Model file for the job. Use its own axes, mm. Face numbers are marked on the shaded views. Coordinates: 2 decimals unless noted, no trailing zeros. Write each loop counter-clockwise with the first axis right and the second up, starting at its lowest first coordinate (ties: lowest second). Pieces come first, ordered by that corner, then holes. Notation, with made-up numbers: M 0,46 L 21,46 A27 cw 21,62 Z; hole C 86,4.25 d4. An arc over 180 degrees is marked long. Put each result on its own line as item: value. Start each with the question number.
Q1. Cut at B-B (y = 21.5). Write the cut outline in (x, z).
Q2. Drop flat-ended pins along their axis: pin 1 (10 mm diameter, centred on y = 10.5, z = -65, fed in from +X); pin 2 (5 mm diameter, centred on x = 0.5, z = -72, fed in from +Y). Give the stop position or say it passes through.
Q3. Pull direction X, two halves, no side cores. Call the marked faces 1, 2 and 3: pulls with the +X half, pulls with the -X half, needs draft (parallel to the pull), parting line crosses it, or undercut.
Q4. Cut at C-C (x = -4). Write the cut outline in (y, z).
Q5. Cut at A-A (z = -57). Write the cut outline in (x, y).
Q6. Drill centre lines: line 1 along X through (y, z) = (9, -53); line 2 along Y through (x, z) = (1, -37); line 3 along X through (y, z) = (2, -64.5). Where is each one in solid material? Low to high.
Q7. Cut at D-D (z = -47.5). Write the cut outline in (x, y).
Autodesk Inventor part; units mm, degrees
ref_plane "YZ Plane" through (0, 0, 0) normal (1, 0, 0) x (0, 1, 0)
ref_plane "XZ Plane" through (0, 0, 0) normal (0, 1, 0) x (-1, 0, 0)
ref_plane "XY Plane" through (0, 0, 0) normal (0, 0, 1) x (1, 0, 0)
sketch "Base" plane through (0, 0, 0) normal (0, 1, 0) x (-1, 0, 0)
  line L0 (-10.6945, -30.7069) -> (-10.6945, -77.3796)
  line L1 (5.3055, -77.3796) -> (5.3055, -30.7069)
  line L2 (5.3055, -30.7069) -> (-10.6945, -30.7069)
  line L3 (5.3055, -77.3796) -> (-10.6945, -77.3796)
  point P0 (0, 0)
extrude "Extrusion1" add sketch "Base" along normal blind 3
sketch "FrontWall" plane through (0, 3, 0) normal (0, 1, 0) x (1, 0, 0)
  line L0 (-5.3055, 77.3796) -> (-5.3055, 30.7069)
  line L1 (-2.7655, 31.0004) -> (-2.7655, 77.0861)
  line L2 (-5.3055, 77.3796) -> (-2.7655, 77.3796)
  line L3 (10.6945, 77.3796) -> (-5.3055, 77.3796)
  line L4 (-2.7655, 77.0861) -> (-2.7655, 77.2936)
  line L5 (-2.7655, 77.2936) -> (-2.7655, 77.3796)
  line L6 (-2.7655, 31.0004) -> (-2.7655, 30.7069)
  line L7 (-5.3055, 30.7069) -> (-2.7655, 30.7069)
  line L8 (-5.3055, 30.7069) -> (10.6945, 30.7069)
  point P0 (0, 0)
extrude "Extrusion2" add sketch "FrontWall" along normal blind 29.464
sketch "Sketch5" plane through (-5.3055, 0, -77.3796) normal (-1, 0, 0) x (0, 0, 1)
  line L0 (-47.9308, 0) -> (-47.9308, 32.464)
  line L1 (0, 0) -> (0, 32.464)
  line L2 (46.1641, 31.6804) -> (0.7141, 31.6804)
  line L3 (0.7141, 31.6804) -> (0.7141, 10.0772)
  line L4 (0.7141, 10.0772) -> (46.1641, 10.0772)
  line L5 (46.1641, 10.0772) -> (46.1641, 31.6804)
  line L6 (23.4391, 30.4798) -> (18.3891, 30.4798)
  line L7 (18.3891, 30.4798) -> (18.3891, 25.6172)
  line L8 (18.3891, 25.6172) -> (28.4983, 25.6172)
  line L9 (28.4983, 25.6172) -> (28.4983, 30.4798)
  line L10 (28.4983, 30.4798) -> (23.4391, 30.4798)
  point P0 (77.3796, 0)
  point P1 (74.13, 0)
  point P2 (10.7141, 20.3272)
  point P3 (36.1565, 20.3272)
  dimension "d27" = 47.9308
  dimension "d28" = 45.45
hole "Hole2" at (-5.3055, 20.3272, -41.2231) at (-5.3055, 20.3272, -66.6655) direction (1, 0, 0) diameter 17.5 end through all
extrude "Extrusion4" cut sketch "Sketch5" against normal blind 29.464 contours L10 L9 L8 L7 L6
fillet "Fillet1" radius 1.27 4 edges at (-4.0355, 30.4798, -58.9905) (-4.0355, 25.6172, -58.9905) (-4.0355, 30.4798, -48.8813) (-4.0355, 25.6172, -48.8813)
fillet "Fillet2" radius 1.27 4 edges at (-4.0355, 32.464, -30.7069) (-4.0355, 32.464, -77.3796) (10.6945, 1.5, -30.7069) (10.6945, 1.5, -77.3796)
sketch "Sketch8" plane through (0, 3, 0) normal (0, 1, 0) x (1, 0, 0)
  line L0 (3.818, 31.9431) -> (4.786, 31.9431)
  line L1 (5.802, 32.9591) -> (5.802, 75.143)
  line L2 (4.786, 76.159) -> (3.818, 76.159)
  line L3 (2.802, 75.143) -> (2.802, 32.9591)
  arc A0 (3.818, 76.159) -> (2.802, 75.143) centre (3.818, 75.143) ccw
  arc A1 (5.802, 75.143) -> (4.786, 76.159) centre (4.786, 75.143) ccw
  arc A2 (2.802, 32.9591) -> (3.818, 31.9431) centre (3.818, 32.9591) ccw
  arc A3 (4.786, 31.9431) -> (5.802, 32.9591) centre (4.786, 32.9591) ccw
  point P0 (0, 0)
  point P1 (5.802, 76.159)
  point P2 (2.802, 76.159)
  dimension "d62" = 3
  dimension "d63" = 1.016
extrude "Extrusion6" cut sketch "Sketch8" against normal through all
properties part number "UltrasonicSensorMountSingle"
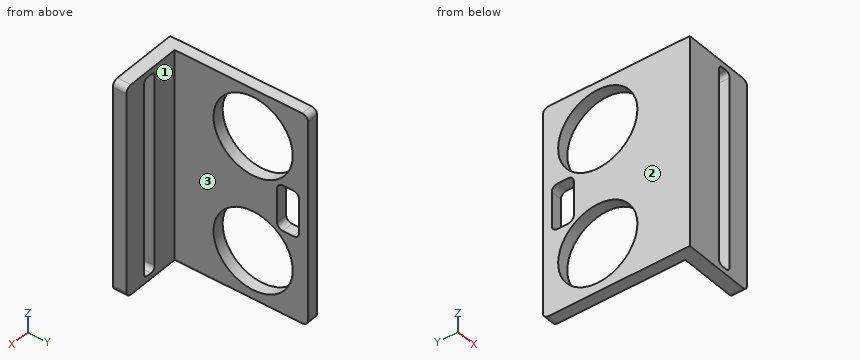
Computed values:
1. outline: M -5.31,-77.38 L -2.77,-77.38 L -2.77,-75.34 L -5.31,-75.34 Z; M -5.31,-57.99 L -2.77,-57.99 L -2.77,-49.89 L -5.31,-49.89 Z; M -5.31,-32.55 L -2.77,-32.55 L -2.77,-30.71 L -5.31,-30.71 Z
2. pin 1: x = -2.77
2. pin 2: y = 3
3. face 1: needs draft
3. face 2: pulls with the -X half
3. face 3: pulls with the +X half
4. outline: M 0,-77.38 L 31.19,-77.38 A1.27 ccw 32.46,-76.11 L 32.46,-31.98 A1.27 ccw 31.19,-30.71 L 0,-30.71 Z; hole C 20.33,-66.67 d17.5; hole C 20.33,-41.22 d17.5; hole M 25.62,-57.72 A1.27 ccw 26.89,-58.99 L 29.21,-58.99 A1.27 ccw 30.48,-57.72 L 30.48,-50.15 A1.27 ccw 29.21,-48.88 L 26.89,-48.88 A1.27 ccw 25.62,-50.15 Z
5. outline: M -5.31,0 L 2.8,0 L 2.8,3 L -2.77,3 L -2.77,25.62 L -5.31,25.62 Z; M -5.31,30.48 L -2.77,30.48 L -2.77,32.46 L -5.31,32.46 Z; M 5.8,0 L 10.69,0 L 10.69,3 L 5.8,3 Z
6. line 1: -5.31 to -2.77
6. line 2: 0 to 3
6. line 3: -5.31 to 2.8, 5.8 to 10.69
7. outline: M -5.31,0 L 2.8,0 L 2.8,3 L -2.77,3 L -2.77,14.23 L -5.31,14.23 Z; M -5.31,26.42 L -2.77,26.42 L -2.77,32.46 L -5.31,32.46 Z; M 5.8,0 L 10.69,0 L 10.69,3 L 5.8,3 Z
